Could you check a few things on this model? Use its own coordinates, in mm. A direction names the side the tool comes from. Give positions to 0.01 mm unless a question says otherwise; leave off trailing zeros. Write each loop counter-clockwise with the first axis right and the second up, starting at its lowest first coordinate (ties: lowest second). Pieces come first, ordered by that corner, then holes. Notation, with made-up numbers: (25.25, 49.5) - (75.25, 49.5) arc R12 ccw to (75.25, 63.5) - close; hole circle Ø7 at (31.25, 77). An arc over 180 degrees is marked (long way). Write item = value, one per line.
from build123d import *

# Parameters (mm, degrees)
F0_R     = 17.9
F1_DEPTH = 53
F2_R     = 5
F3_DEPTH = 1
F4_R     = 1.575
F5_DEPTH = 10
F6_W     = 9.9145695567
F6_H     = 3.6825537682
F7_DEPTH = 3
F9_DEPTH = 2


with BuildPart() as f1:
    # F0 (on Front) → F1 (new body)
    with BuildSketch(Plane.XZ):
        with Locations((-27.1942447871, 20.9622308612)):
            Circle(F0_R)
    extrude(amount=F1_DEPTH)

    # F2 (on face) → F3 (join)
    with BuildSketch(Plane(origin=(0, 0, 0), x_dir=(-1, 0, 0), z_dir=(0, 1, 0))):
        with Locations((27.1942447871, 20.9622308612)):
            Circle(F2_R)
    extrude(amount=F3_DEPTH)

    # F4 (on face) → F5 (join)
    with BuildSketch(Plane(origin=(0, 1, 0), x_dir=(-1, 0, 0), z_dir=(0, 1, 0))):
        with Locations((27.1942447871, 20.9622308612)):
            Circle(F4_R)
    extrude(amount=F5_DEPTH)

    # F6 (on face) → F7 (cut)
    with BuildSketch(Plane.XZ.offset(53)):
        with Locations((-26.6985148191, 27.265066281)):
            Rectangle(F6_W, F6_H)
    extrude(amount=-F7_DEPTH, mode=Mode.SUBTRACT)

    # F8 (on face) → F9 (join)
    with BuildSketch(Plane.XZ.offset(53)):
        with BuildLine():
            Line((-35.4207989488, 42.9829595067), (-35.4207989488, 36.8598346626))
            ThreePointArc((-35.4207989488, 36.8598346626), (-33.3154303096, 37.7830836279), (-31.1090964824, 38.428882979))
            Line((-31.1090964824, 38.428882979), (-31.1090964824, 42.9829595067))
            Line((-31.1090964824, 42.9829595067), (-35.4207989488, 42.9829595067))
        make_face()
        with BuildLine():
            Line((-29.0810409933, 42.9829595067), (-29.0810409933, 38.76251176))
            ThreePointArc((-29.0810409933, 38.76251176), (-26.7457383718, 38.8566110403), (-24.4180820882, 38.6456389227))
            Line((-24.4180820882, 38.6456389227), (-24.4180820882, 42.9829595067))
            Line((-24.4180820882, 42.9829595067), (-29.0810409933, 42.9829595067))
        make_face()
        with BuildLine():
            ThreePointArc((-22.4494244903, 38.2219145301), (-20.5451738039, 37.5814924291), (-18.7246836722, 36.7317119725))
            Line((-18.7246836722, 36.7317119725), (-18.7246836722, 42.9829595067))
            Line((-18.7246836722, 42.9829595067), (-22.4494244903, 42.9829595067))
            Line((-22.4494244903, 42.9829595067), (-22.4494244903, 38.2219145301))
        make_face()
    extrude(amount=-F9_DEPTH)


solid = f1.part
1. If we section it at D-D, the plane x = -38.5: Please give me the cut outline in (y, z), and give its area (3 significant figures).
Filled sheet:
outline = (-53, 7.08) - (0, 7.08) - (0, 34.84) - (-53, 34.84) - close
area = 1,470 mm2
2. For pin 1 (1 mm diameter, centred on x = -24.5, y = -24.5, fed in from +Z); pin 2 (2 mm diameter, centred on y = -52, z = 40.5, fed in from +X); pin 3 (2.5 mm diameter, centred on y = -52, z = 28, fed in from -X), each with a flat end and sliding along its axis, tell me the tip position at first contact or that it passes through.
Filled sheet:
pin_1 = 38.73
pin_2 = -18.72
pin_3 = -44.13
3. Which directions (+Z, -Z, +X, -X, +Y, -Y) give clear straight access to the entire face, cutting with the end or side of a thin tool? Please do faces 1 (the face through (-24.418, -52, 41)), 2 (the face through (-27, -52, 29.106)), 3 (the face through (-21, -51, 41)), 4 (the face through (-35.421, -52, 40)), 5 (the face through (-28.697, 5.93, 21.435)).
Filled sheet:
face_1 = +Z, +Y, -Y
face_2 = -Y
face_3 = +Z, +X, +Y
face_4 = +Z, -X, +Y, -Y
face_5 = +Y
4. If we section it at A-A, the plane z = 24.5: Please give me the cut outline in (x, y), and give its area (3 significant figures).
Filled sheet:
outline = (-44.74, -53) - (-9.65, -53) - (-9.65, 0) - (-23.66, 0) - (-23.66, 1) - (-30.73, 1) - (-30.73, 0) - (-44.74, 0) - close
area = 1,870 mm2
5. If we section it at B-B, the plane x = -30: Please give me the cut outline in (y, z), and give its area (3 significant figures).
Filled sheet:
outline = (-53, 3.28) - (0, 3.28) - (0, 16.82) - (1, 16.82) - (1, 25.1) - (0, 25.1) - (0, 38.64) - (-53, 38.64) - (-53, 29.11) - (-50, 29.11) - (-50, 25.42) - (-53, 25.42) - close
area = 1,870 mm2
6. I need wall thicknesses on line 1 (Y direction, x = -26, z = 5.5); line 2 (X direction, y = -36, z = 12.5); line 3 (X direction, y = -42, z = 23.5). Which ranges of each line are inside material? Lowest first, please.
Filled sheet:
line_1 = -53 to 0
line_2 = -42.97 to -11.42
line_3 = -44.91 to -9.48
7. Thinking about a two-plate mould opening in X: for faces 6 (the face through (-23, 0, 17)), 7 (the face through (-29.081, -52, 41)), 8 (the face through (-18.725, -52, 40)), which applies, pulls with the +X half, pulls with the -X half, needs draft (parallel to the pull), parting line crosses it, or undercut?
Filled sheet:
face_6 = needs draft
face_7 = undercut
face_8 = pulls with the +X half
8. If we section it at C-C, the plane y = -10: Please give me the cut outline in (x, z).
Filled sheet:
outline = circle Ø35.8 at (-27.19, 20.96)
